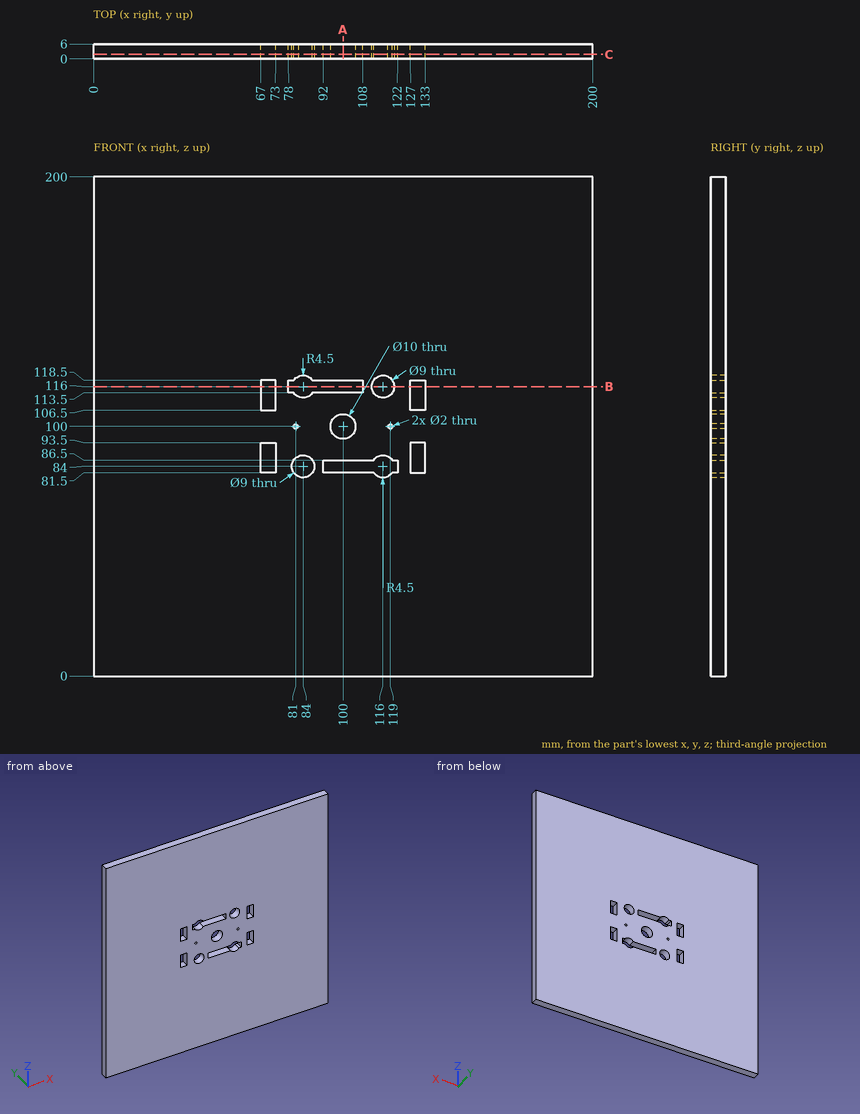
Could you check a few things on this drawing? It's one solid part, dimensions in mm from its lowest x, y, z. Give positions to 0.01 mm unless a question says otherwise; leave off trailing zeros. Loops run counter-clockwise (first coordinate to the right, second up) from the corner with the lowest first, then second, coordinate; pieces in that order, holes last. Notation, with made-up numbers: M 5,80.25 L 28,80.25 A15 ccw 28,105.25 Z; hole C 27.5,40 d8. An arc over 180 degrees is marked long. Answer as a JSON object with one key per item and string values.
Q1. Suppose I cut it at B-B, the plane z = 116. List the corners of the cut face in (x, y) for me, plus the area to 3 significant figures.
Values found:
{"outline": "M 0,0 L 67,0 L 67,6 L 0,6 Z; M 73,0 L 78,0 L 78,6 L 73,6 Z; M 108,0 L 111.5,0 L 111.5,6 L 108,6 Z; M 120.5,0 L 127,0 L 127,6 L 120.5,6 Z; M 133,0 L 200,0 L 200,6 L 133,6 Z", "area": "894 mm²"}
Q2. Suppose I cut it at C-C, the plane y = 1.8. State how many separate pieces and enclosed holes the cut face has, plus the area to 3 significant figures.
Values found:
{"separate pieces": "1", "enclosed holes": "11", "area": "39,200 mm²"}
Q3. Suppose I cut it at A-A, the plane x = 100. List the corners of the cut face in (y, z) for me, plus the area to 3 significant figures.
Values found:
{"outline": "M 0,0 L 6,0 L 6,81.5 L 0,81.5 Z; M 0,86.5 L 6,86.5 L 6,95 L 0,95 Z; M 0,105 L 6,105 L 6,113.5 L 0,113.5 Z; M 0,118.5 L 6,118.5 L 6,200 L 0,200 Z", "area": "1,080 mm²"}
Q4. For P1, Ø7, axis at x = 116, z = 116, coming from the -Y side; P2, Ø4, axis at x = 77.5, z = 176.5, coming from the -Y side, each with a flat end and sliding along its axis, tell me the tip position at first contact or that it passes through.
Values found:
{"P1": "passes through", "P2": "stops at y = 0"}
Q5. If I drill on probe 1 along Z at (x, y) = (105.5, 4.6); probe 2 along Z at (x, y) = (116, 2.45); probe 3 along X at (y, z) = (5.25, 107.5), over which ranges is the centre line in solid material (lowest first)? Write a range as [from, to].
Values found:
{"probe 1": "z = [0, 81.5], [86.5, 113.5], [118.5, 200]", "probe 2": "z = [0, 79.5], [88.5, 111.5], [120.5, 200]", "probe 3": "x = [0, 67], [73, 127], [133, 200]"}
